Autodesk Fusion 360 part; units mm, degrees
sketch "スケッチ1" plane through (0, 0, 0) normal (0, 1, 0) x (1, 0, 0)
  line L0 (8, 10) -> (-8, 10)
  line L1 (-10, 8) -> (-10, -8)
  line L2 (-8, -10) -> (8, -10)
  line L3 (10, -8) -> (10, 8)
  line L4 (10, 10) -> (-10, -10) construction
  line L5 (-10, 10) -> (10, -10) construction
  circle A0 centre (0, 0) radius 2.6
  line L6 (-3.2, -10) -> (-3.2, -8.65)
  line L7 (-3.2, -8.65) -> (-4.6, -8.65)
  line L8 (-5.1, -8.15) -> (-5.1, -6.3678)
  line L9 (-4.9536, -6.0142) -> (-3.4251, -4.4858)
  line L10 (0, 0) -> (0, -10) construction
  line L11 (-2.0109, -3.9) -> (0, -3.9)
  arc A1 (-5.1, -8.15) -> (-4.6, -8.65) centre (-4.6, -8.15) ccw
  arc A2 (-4.9536, -6.0142) -> (-5.1, -6.3678) centre (-4.6, -6.3678) ccw
  arc A3 (-2.0109, -3.9) -> (-3.4251, -4.4858) centre (-2.0109, -5.9) ccw
  arc A4 (-10, -8) -> (-8, -10) centre (-8, -8) ccw
  arc A5 (10, 8) -> (8, 10) centre (8, 8) ccw
  arc A6 (8, -10) -> (10, -8) centre (8, -8) ccw
  arc A7 (-8, 10) -> (-10, 8) centre (-8, 8) ccw
  line L12 (3.2, -10) -> (3.2, -8.65)
  line L13 (3.2, -8.65) -> (4.6, -8.65)
  arc A8 (4.6, -8.65) -> (5.1, -8.15) centre (4.6, -8.15) ccw
  line L14 (5.1, -8.15) -> (5.1, -6.3678)
  arc A9 (5.1, -6.3678) -> (4.9536, -6.0142) centre (4.6, -6.3678) ccw
  line L15 (4.9536, -6.0142) -> (3.4251, -4.4858)
  arc A10 (3.4251, -4.4858) -> (2.0109, -3.9) centre (2.0109, -5.9) ccw
  line L16 (2.0109, -3.9) -> (0, -3.9)
  line L17 (10, -3.2) -> (8.65, -3.2)
  line L18 (8.65, -3.2) -> (8.65, -4.6)
  arc A11 (8.15, -5.1) -> (8.65, -4.6) centre (8.15, -4.6) ccw
  line L19 (8.15, -5.1) -> (6.3678, -5.1)
  arc A12 (6.0142, -4.9536) -> (6.3678, -5.1) centre (6.3678, -4.6) ccw
  line L20 (6.0142, -4.9536) -> (4.4858, -3.4251)
  arc A13 (3.9, -2.0109) -> (4.4858, -3.4251) centre (5.9, -2.0109) ccw
  line L21 (3.9, -2.0109) -> (3.9, 0)
  line L22 (3.9, 2.0109) -> (3.9, 0)
  arc A14 (4.4858, 3.4251) -> (3.9, 2.0109) centre (5.9, 2.0109) ccw
  line L23 (6.0142, 4.9536) -> (4.4858, 3.4251)
  arc A15 (6.3678, 5.1) -> (6.0142, 4.9536) centre (6.3678, 4.6) ccw
  line L24 (8.15, 5.1) -> (6.3678, 5.1)
  arc A16 (8.65, 4.6) -> (8.15, 5.1) centre (8.15, 4.6) ccw
  line L25 (8.65, 3.2) -> (8.65, 4.6)
  line L26 (10, 3.2) -> (8.65, 3.2)
  line L27 (3.2, 10) -> (3.2, 8.65)
  line L28 (3.2, 8.65) -> (4.6, 8.65)
  arc A17 (5.1, 8.15) -> (4.6, 8.65) centre (4.6, 8.15) ccw
  line L29 (5.1, 8.15) -> (5.1, 6.3678)
  arc A18 (4.9536, 6.0142) -> (5.1, 6.3678) centre (4.6, 6.3678) ccw
  line L30 (4.9536, 6.0142) -> (3.4251, 4.4858)
  arc A19 (2.0109, 3.9) -> (3.4251, 4.4858) centre (2.0109, 5.9) ccw
  line L31 (2.0109, 3.9) -> (0, 3.9)
  line L32 (-2.0109, 3.9) -> (0, 3.9)
  arc A20 (-3.4251, 4.4858) -> (-2.0109, 3.9) centre (-2.0109, 5.9) ccw
  line L33 (-4.9536, 6.0142) -> (-3.4251, 4.4858)
  arc A21 (-5.1, 6.3678) -> (-4.9536, 6.0142) centre (-4.6, 6.3678) ccw
  line L34 (-5.1, 8.15) -> (-5.1, 6.3678)
  arc A22 (-4.6, 8.65) -> (-5.1, 8.15) centre (-4.6, 8.15) ccw
  line L35 (-3.2, 8.65) -> (-4.6, 8.65)
  line L36 (-3.2, 10) -> (-3.2, 8.65)
  line L37 (-10, 3.2) -> (-8.65, 3.2)
  line L38 (-8.65, 3.2) -> (-8.65, 4.6)
  arc A23 (-8.15, 5.1) -> (-8.65, 4.6) centre (-8.15, 4.6) ccw
  line L39 (-8.15, 5.1) -> (-6.3678, 5.1)
  arc A24 (-6.0142, 4.9536) -> (-6.3678, 5.1) centre (-6.3678, 4.6) ccw
  line L40 (-6.0142, 4.9536) -> (-4.4858, 3.4251)
  arc A25 (-3.9, 2.0109) -> (-4.4858, 3.4251) centre (-5.9, 2.0109) ccw
  line L41 (-3.9, 2.0109) -> (-3.9, 0)
  line L42 (-3.9, -2.0109) -> (-3.9, 0)
  arc A26 (-4.4858, -3.4251) -> (-3.9, -2.0109) centre (-5.9, -2.0109) ccw
  line L43 (-6.0142, -4.9536) -> (-4.4858, -3.4251)
  arc A27 (-6.3678, -5.1) -> (-6.0142, -4.9536) centre (-6.3678, -4.6) ccw
  line L44 (-8.15, -5.1) -> (-6.3678, -5.1)
  arc A28 (-8.65, -4.6) -> (-8.15, -5.1) centre (-8.15, -4.6) ccw
  line L45 (-8.65, -3.2) -> (-8.65, -4.6)
  line L46 (-10, -3.2) -> (-8.65, -3.2)
  dimension "d1" = 20
  dimension "d2" = 20
  dimension "d3" = 5.2
  dimension "d4" = 1.35
  dimension "d5" = 3.2
  dimension "d6" = 5.1
  dimension "d7" = 6.1
  dimension "d8" = 0.75
  dimension "d9" = 0.5
  dimension "d10" = 2
  dimension "d11" = 2
  dimension "d12" = 2
  dimension "d13" = 2
  dimension "d14" = 2
  dimension "d16" = 360
extrude "押し出し1" add sketch "スケッチ1" along normal mid plane 310 contours L0 L1 L2 L3 L6 L7 L8 L9 L11 A1 A2 A3 A4 A5 A6 A7 L12 L13 A8 L14 A9 L15 A10 L16 L17 L18 A11 L19 A12 L20 A13 L21 L22 A14 L23 A15 L24 A16 L25 L26 L27 L28 A17 L29 A18 L30 A19 L31 L32 A20 L33 A21 L34 A22 L35 L36 L37 L38 A23 L39 A24 L40 A25 L41 L42 A26 L43 A27 L44 A28 L45 L46
Could you check a few things on this model? Use its own coordinates, in mm. Give positions to 0.01 mm unless a question says otherwise; leave off trailing zeros. Answer in a Markdown table with one row per item. Add a question column.
Item 1: I'm going to push flat-ended pins straight in: P1, Ø1.5, axis at x = -9.5, y = -6.5, coming from the -Z side; P2, Ø4, axis at y = 95, z = 1, coming from the +X side; P3, Ø1.5, axis at x = 9, y = -14.5, coming from the -Z side; P4, Ø4, axis at x = -2.5, z = 4, coming from the +Y side. Where does each tip first touch, or does it pass through?
Item 2: We'd pull the mould along Z, two halves only. Please class faces 1 (the cylindrical face through (-0.338, -2.17, 2.578)), 2 (the flat face through (-6, -2, -10)), 3 (the flat face through (10, -2, 6)): pulls with the +Z half, pulls with the -Z half, needs draft (parallel to the pull), parting line crosses it, or undercut.
Item 3: Please list where these lines run through material, in increasing order: probe 1 along X at (y, z) = (90, 0); probe 2 along Z at (x, y) = (5.5, -71); probe 3 along Z at (x, y) = (-8, -86).
Result:
| question | item | result |
|---|---|---|
| 1 | P1 | z = -9.85 |
| 1 | P2 | x = 4.16 |
| 1 | P3 | z = -9.98 |
| 1 | P4 | y = 155 |
| 2 | face 1 | undercut |
| 2 | face 2 | pulls with the -Z half |
| 2 | face 3 | needs draft |
| 3 | probe 1 | -3.9 to -2.6, 2.6 to 3.9 |
| 3 | probe 2 | -10 to -4.44, 4.44 to 10 |
| 3 | probe 3 | -10 to -5.1, 5.1 to 10 |
